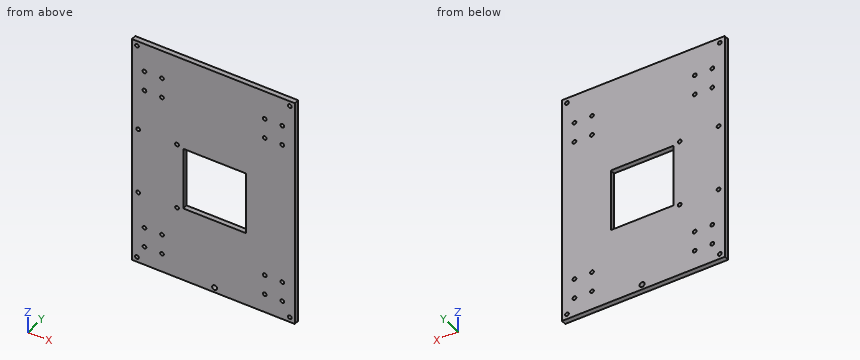
from build123d import *

# Parameters (mm, degrees)
SKETCH1_W           = 130
SKETCH1_H           = 185
SKETCH1_R           = 1.5
BOSS_EXTRUDE1_DEPTH = 4
SKETCH2_W           = 50
SKETCH2_H           = 50
CUT_EXTRUDE1_DEPTH  = 4
SKETCH3_R           = 1.5
CUT_EXTRUDE2_DEPTH  = 49.5
SKETCH4_R           = 2
CUT_EXTRUDE3_DEPTH  = 49.5
SKETCH5_R           = 1.5
CUT_EXTRUDE5_DEPTH  = 10


with BuildPart() as part:
    # Sketch1 → Boss-Extrude1 (new body)
    with BuildSketch(Plane(origin=(0, 0, 0), x_dir=(1, 0, 0), z_dir=(0, 1, 0))):
        with Locations((65, 92.5)):
            Rectangle(SKETCH1_W, SKETCH1_H)
        with Locations(Location((10, 39, 0), (0, 0, 270))):
            Circle(SKETCH1_R, mode=Mode.SUBTRACT)
        with Locations(Location((24, 39, 0), (0, 0, 270))):
            Circle(SKETCH1_R, mode=Mode.SUBTRACT)
        with Locations(Location((10, 23, 0), (0, 0, 270))):
            Circle(SKETCH1_R, mode=Mode.SUBTRACT)
        with Locations(Location((24, 23, 0), (0, 0, 270))):
            Circle(SKETCH1_R, mode=Mode.SUBTRACT)
        with Locations(Location((120, 23, 0), (0, 0, 90))):
            Circle(SKETCH1_R, mode=Mode.SUBTRACT)
        with Locations(Location((120, 39, 0), (0, 0, 90))):
            Circle(SKETCH1_R, mode=Mode.SUBTRACT)
        with Locations(Location((106, 39, 0), (0, 0, 90))):
            Circle(SKETCH1_R, mode=Mode.SUBTRACT)
        with Locations(Location((106, 23, 0), (0, 0, 90))):
            Circle(SKETCH1_R, mode=Mode.SUBTRACT)
        with Locations(Location((106, 170, 0), (0, 0, 270))):
            Circle(SKETCH1_R, mode=Mode.SUBTRACT)
        with Locations(Location((120, 170, 0), (0, 0, 270))):
            Circle(SKETCH1_R, mode=Mode.SUBTRACT)
        with Locations(Location((106, 154, 0), (0, 0, 270))):
            Circle(SKETCH1_R, mode=Mode.SUBTRACT)
        with Locations(Location((120, 154, 0), (0, 0, 270))):
            Circle(SKETCH1_R, mode=Mode.SUBTRACT)
        with Locations(Location((24, 154, 0), (0, 0, 90))):
            Circle(SKETCH1_R, mode=Mode.SUBTRACT)
        with Locations(Location((24, 170, 0), (0, 0, 90))):
            Circle(SKETCH1_R, mode=Mode.SUBTRACT)
        with Locations(Location((10, 170, 0), (0, 0, 90))):
            Circle(SKETCH1_R, mode=Mode.SUBTRACT)
        with Locations(Location((10, 154, 0), (0, 0, 90))):
            Circle(SKETCH1_R, mode=Mode.SUBTRACT)
    extrude(amount=BOSS_EXTRUDE1_DEPTH)

    # Sketch2 → Cut-Extrude1 (cut)
    with BuildSketch(Plane(origin=(0, 4, 0), x_dir=(1, 0, 0), z_dir=(0, 1, 0))):
        with Locations((66, 100)):
            Rectangle(SKETCH2_W, SKETCH2_H)
    extrude(amount=-CUT_EXTRUDE1_DEPTH, mode=Mode.SUBTRACT)

    # Sketch3 → Cut-Extrude2 (cut)
    with BuildSketch(Plane(origin=(0, 4, 0), x_dir=(1, 0, 0), z_dir=(0, 1, 0))):
        with Locations(Location((126, 4, 0), (0, 0, 270))):
            Circle(SKETCH3_R)
        with Locations(Location((126, 181, 0), (0, 0, 90))):
            Circle(SKETCH3_R)
        with Locations(Location((4, 4, 0), (0, 0, 90))):
            Circle(SKETCH3_R)
        with Locations(Location((4, 181, 0), (0, 0, 270))):
            Circle(SKETCH3_R)
    extrude(amount=-CUT_EXTRUDE2_DEPTH, mode=Mode.SUBTRACT)

    # Sketch4 → Cut-Extrude3 (cut)
    with BuildSketch(Plane(origin=(0, 4, 0), x_dir=(1, 0, 0), z_dir=(0, 1, 0))):
        with Locations(Location((66, 181, 0), (0, 0, 90))):
            Circle(SKETCH4_R)
    extrude(amount=-CUT_EXTRUDE3_DEPTH, mode=Mode.SUBTRACT)

    # Sketch5 → Cut-Extrude5 (cut)
    with BuildSketch(Plane(origin=(0, 4, 0), x_dir=(1, 0, 0), z_dir=(0, 1, 0))):
        with Locations(Location((5, 126.5, 0), (0, 0, 270))):
            Circle(SKETCH5_R)
        with Locations(Location((5, 73.5, 0), (0, 0, 90))):
            Circle(SKETCH5_R)
        with Locations(Location((36, 126.5, 0), (0, 0, 90))):
            Circle(SKETCH5_R)
        with Locations(Location((36, 73.5, 0), (0, 0, 270))):
            Circle(SKETCH5_R)
    extrude(amount=-CUT_EXTRUDE5_DEPTH, mode=Mode.SUBTRACT)


solid = part.part
Geometry: final body of the model. Coordinates: model frame, mm. Round coordinates to 2 decimals unless told otherwise and drop trailing zeros.
Q1. Pin query (flat end, axial travel): pin 1 (2.5 mm diameter, centred on x = 4, z = -4, fed in from -Y). Return the tip coordinate at first contact, or that it passes through.
Result sheet:
pin 1: passes through
Q2. Material intervals for probe 1 along Z at (x, y) = (126, 2.75); probe 2 along Z at (x, y) = (120, 1.4); probe 3 along X at (y, z) = (1.65, -181), sorted ascending.
Result sheet:
probe 1: z = -185 to -182.5, -179.5 to -5.5, -2.5 to 0
probe 2: z = -185 to -171.5, -168.5 to -155.5, -152.5 to -40.5, -37.5 to -24.5, -21.5 to 0
probe 3: x = 0 to 2.5, 5.5 to 64, 68 to 124.5, 127.5 to 130
Q3. Section A-A, the plane y = 1.45. Give the number of separate pieces and of enclosed holes in the cut face, and give its area (3 significant figures).
Result sheet:
separate pieces: 1
enclosed holes: 26
area: 21,400 mm2
